from build123d import *

# Parameters (mm, degrees)
ESQUISSE1_R             = 52.5
BOSS_EXTRU_1_DEPTH      = 10
ESQUISSE2_R             = 52.5
BOSS_EXTRU_2_DEPTH      = 3
ENL_V_START             = -3
ESQUISSE3_R             = 2.75
ENL_V_MAT_EXTRU_2_DEPTH = 73.375725535
ESQUISSE4_R             = 1.55
ENL_V_MAT_EXTRU_3_DEPTH = 76.375725535


with BuildPart() as part:
    # Esquisse1 → Boss.-Extru.1 (new body)
    with BuildSketch(Plane(origin=(0, 0, 0), x_dir=(1, 0, 0), z_dir=(0, 1, 0))):
        with Locations(Location((0, 0, 0), (0, 0, 270))):
            Circle(ESQUISSE1_R)
        with BuildLine():
            ThreePointArc((-4, 47.5), (0, 43.5), (4, 47.5))
            Line((4, 47.5), (4, 48.127435003))
            ThreePointArc((4, 48.127435003), (4.676150568, 49.626575651), (6.24742268, 50.112071498))
            ThreePointArc((6.24742268, 50.112071498), (43.734282891, 25.25), (46.522038294, -19.645609))
            ThreePointArc((46.522038294, -19.645609), (45.3159505, -20.763622642), (43.679581332, -20.599615887))
            Line((43.679581332, -20.599615887), (43.13620668, -20.285898385))
            ThreePointArc((43.13620668, -20.285898385), (37.672105065, -21.75), (39.13620668, -27.214101615))
            Line((39.13620668, -27.214101615), (39.679581332, -27.527819117))
            ThreePointArc((39.679581332, -27.527819117), (40.639799932, -28.862953009), (40.274615614, -30.466462499))
            ThreePointArc((40.274615614, -30.466462499), (0, -50.5), (-40.274615614, -30.466462499))
            ThreePointArc((-40.274615614, -30.466462499), (-40.639799932, -28.862953009), (-39.679581332, -27.527819117))
            Line((-39.679581332, -27.527819117), (-39.13620668, -27.214101615))
            ThreePointArc((-39.13620668, -27.214101615), (-37.672105065, -21.75), (-43.13620668, -20.285898385))
            Line((-43.13620668, -20.285898385), (-43.679581332, -20.599615887))
            ThreePointArc((-43.679581332, -20.599615887), (-45.3159505, -20.763622642), (-46.522038294, -19.645609))
            ThreePointArc((-46.522038294, -19.645609), (-43.734282891, 25.25), (-6.24742268, 50.112071498))
            ThreePointArc((-6.24742268, 50.112071498), (-4.676150568, 49.626575651), (-4, 48.127435003))
            Line((-4, 48.127435003), (-4, 47.5))
        make_face(mode=Mode.SUBTRACT)
    extrude(amount=BOSS_EXTRU_1_DEPTH)

    # Esquisse2 → Boss.-Extru.2 (add)
    with BuildSketch(Plane(origin=(0, 10, 0), x_dir=(1, 0, 0), z_dir=(0, 1, 0))):
        with Locations(Location((0, 0, 0), (0, 0, 270))):
            Circle(ESQUISSE2_R)
    extrude(amount=BOSS_EXTRU_2_DEPTH)

    # Esquisse3 → Enlèv. mat.-Extru.2 (cut, through all)
    with BuildSketch(Plane.XZ.offset(ENL_V_START)):
        with Locations(Location((0, -47.5, 0), (0, 0, 270))):
            Circle(ESQUISSE3_R)
        with Locations(Location((-41.13620668, 23.75, 0), (0, 0, 270))):
            Circle(ESQUISSE3_R)
        with Locations(Location((41.13620668, 23.75, 0), (0, 0, 270))):
            Circle(ESQUISSE3_R)
    extrude(amount=-ENL_V_MAT_EXTRU_2_DEPTH, mode=Mode.SUBTRACT)

    # Esquisse4 → Enlèv. mat.-Extru.3 (cut, through all)
    with BuildSketch(Plane.XZ):
        with Locations(Location((0, -47.5, 0), (0, 0, 270))):
            Circle(ESQUISSE4_R)
        with Locations(Location((-41.13620668, 23.75, 0), (0, 0, 270))):
            Circle(ESQUISSE4_R)
        with Locations(Location((41.13620668, 23.75, 0), (0, 0, 270))):
            Circle(ESQUISSE4_R)
    extrude(amount=-ENL_V_MAT_EXTRU_3_DEPTH, mode=Mode.SUBTRACT)


solid = part.part
Work out the finished part from the listing and answer in its coordinate system (mm). A direction names the side the tool comes from. Coordinates: 2 decimals unless noted, no trailing zeros. Write each loop counter-clockwise with the first axis right and the second up, starting at its lowest first coordinate (ties: lowest second). Pieces come first, ordered by that corner, then holes. Notation, with made-up numbers: M -8,81.25 L 40,81.25 A12 cw 40,86.25 Z; hole C 71,-8 d5. An arc over 180 degrees is marked long. Answer as CSV lines item,"result". Start each with the question number.
Item 1: Determine the mould class of faces 1 (the face through (15.77, 6.409, 50.076)), 2 (the face through (1, 13, -1)), 3 (the face through (-37.629, 4.93, 21.827)) for opening direction X: released by +X, released by -X, zero draft, split by the parting line, or undercut.
Item 2: Consider L1, parallel to X at y = 1.8, z = 23.75; L2, parallel to X at y = 5, z = 25.5; L3, parallel to Y at x = -9, z = 46. Determine where each line is inside the solid, lowest interval first.
Item 3: Section A-A on x = 0 is taken. Write down the section's boundary in (y, z), and give its area (3 significant figures).
Item 4: Section C-C on z = 23.75 is taken. Write down the section's boundary in (x, y).
Item 5: Section B-B on z = 0 is taken. Write down the section's boundary in (x, y), and give its area (3 significant figures).
Item 6: Flat-ended cylindrical pins translate along their axes: P1, Ø9, axis at x = 0, z = -47.5, coming from the -Y side; P2, Ø5, axis at x = 39.5, y = 7, coming from the -Z side; P3, Ø5, axis at x = 13, z = -10.5, coming from the -Y side; P4, Ø3, axis at x = 0.5, z = -47, coming from the +Y side. Find the tip coordinate at first contact, or state that the pin passes through.
Item 7: A tool of negligible diameter and unlimited length cuts with its end or side. For faces 4 (the face through (0.466, 1.479, -48.978)), 5 (the face through (-41, 3, 22)), 6 (the face through (-40.644, 4.93, 28.886)), from which of +Z, -Z, +X, -X, +Y, -Y can it reach the whole face along a straight path? Write none if from no direction.
Item 8: Section D-D on y = 7.75 is taken. Write down the section's boundary in (x, z), and give its area (3 significant figures).
Checks:
1,face 1,"split by the parting line"
1,face 2,"zero draft"
1,face 3,"undercut"
2,L1,"x = -46.82 to -42.69, -39.59 to -37.14, 37.14 to 39.59, 42.69 to 46.82"
2,L2,"x = -45.89 to -43.26, -39.01 to -37.54, 37.54 to 39.01, 43.26 to 45.89"
2,L3,"y = 10 to 13"
3,outline,"M 0,-52.5 L 13,-52.5 L 13,-50.25 L 3,-50.25 L 3,-49.05 L 0,-49.05 Z; M 0,-45.95 L 3,-45.95 L 3,-44.75 L 13,-44.75 L 13,52.5 L 0,52.5 L 0,50.5 L 10,50.5 L 10,-43.5 L 0,-43.5 Z"
3,area,"361 mm²"
4,outline,"M -46.82,0 L -42.69,0 L -42.69,3 L -43.89,3 L -43.89,13 L -46.82,13 Z; M -39.59,0 L -37.14,0 L -37.14,10 L 37.14,10 L 37.14,0 L 39.59,0 L 39.59,3 L 38.39,3 L 38.39,13 L -38.39,13 L -38.39,3 L -39.59,3 Z; M 42.69,0 L 46.82,0 L 46.82,13 L 43.89,13 L 43.89,3 L 42.69,3 Z"
5,outline,"M -52.5,0 L -50.5,0 L -50.5,10 L 50.5,10 L 50.5,0 L 52.5,0 L 52.5,13 L -52.5,13 Z"
5,area,"355 mm²"
6,P1,"stops at y = 0"
6,P2,"stops at z = -37.25"
6,P3,"stops at y = 10"
6,P4,"stops at y = 3"
7,face 4,"+Y, -Y"
7,face 5,"+Y"
7,face 6,"-Y"
8,outline,"C 0,0 d105; hole M -46.52,19.65 A50.5 ccw -6.25,-50.11 A2 ccw -4,-48.13 L -4,-47.5 A4 cw 4,-47.5 L 4,-48.13 A2 ccw 6.25,-50.11 A50.5 ccw 46.52,19.65 A2 ccw 43.68,20.6 L 43.14,20.29 A4 cw 39.14,27.21 L 39.68,27.53 A2 ccw 40.27,30.47 A50.5 ccw -40.27,30.47 A2 ccw -39.68,27.53 L -39.14,27.21 A4 cw -43.14,20.29 L -43.68,20.6 A2 ccw Z; hole C -41.14,23.75 d5.5; hole C 0,-47.5 d5.5; hole C 41.14,23.75 d5.5"
8,area,"729 mm²"
